Can you work these out from the model? Positions are in its coordinate system, mm. A direction names the side the tool comes from. Coordinates: 2 decimals unless noted, no trailing zeros. Loops run counter-clockwise (first coordinate to the right, second up) from the corner with the lowest first, then second, coordinate; pieces in that order, holes last. Notation, with made-up numbers: (80.25, 69.5) -> (132.25, 69.5) arc R23 ccw to (132.25, 108.5) -> close; hole circle Ø11 at (7.5, -19.75). An arc over 180 degrees is marked (long way). Use one line per item in the form item = value. Start each with the question number.
(1) Imagine slicing it at A-A (x = 0). List the corners of the cut face in (y, z) for me, plus the area to 3 significant figures.
(2) Imagine slicing it at B-B (z = 5). List the corners of the cut face in (x, y) for me.
(3) I need wall thicknesses on line 1 (X direction, y = -6.5, z = 33); line 2 (Z direction, x = 9.25, y = 2); line 3 (Y direction, x = -5, z = 25.5) (3 decimals). Which ranges of each line are inside material? Lowest first, please. Write a range as [from, to].
(4) On a 3-axis mill with a long thin cutter (end or side, diameter ignored), from which of +Z, -Z, +X, -X, +Y, -Y can I reach the whole of each face in a straight line? I mean faces 5 (the flat face through (-2, -9, 38)), 6 (the flat face through (-4, 8, 38)), 7 (the cylindrical face through (5.094, 7.438, 46.381)). Say none if no direction works.
(5) I'm going to push flat-ended pins straight in: pin 1 (2.5 mm diameter, centred on x = 9, y = -2.5, fed in from -Z); pin 2 (4 mm diameter, centred on y = -7.5, z = 5.5, fed in from -X); pin 3 (3 mm diameter, centred on x = 5, z = 23.5, fed in from +Y). Where does each tip first touch, or does it pass through?
(6) Thinking about a two-plate mould opening in X: for faces 1 (the flat face through (4.6, 8.79, 46.38)), 2 (the flat face through (0, 9, 38)), 3 (the cylindrical face through (-6.726, -6.003, 46.381)), 4 (the cylindrical face through (-1.1, -8.9, 46.4)), which applies, released by +X, released by -X, zero draft, split by the parting line, or undercut?
```python
from build123d import *

# Parameters (mm, degrees)
SKETCH1_R           = 8
BOSS_EXTRUDE1_DEPTH = 55
BOSS_EXTRUDE2_START = -17
BOSS_EXTRUDE2_DEPTH = 17
CIRPATTERN1_COUNT   = 13


with BuildPart() as part:
    # Sketch1 → Boss-Extrude1 (new body)
    with BuildSketch(Plane.XY):
        Circle(SKETCH1_R)
    extrude(amount=BOSS_EXTRUDE1_DEPTH)

    # Sketch2 → Boss-Extrude2 (add)
    with BuildSketch(Plane.XY.offset(55).offset(BOSS_EXTRUDE2_START)):
        with BuildLine():
            Line((-0.787121101, 9.92163467), (0.787121101, 9.92163467))
            ThreePointArc((0.787121101, 9.92163467), (1.056170344, 8.938993112), (1.115168142, 7.921893714))
            ThreePointArc((1.115168142, 7.921893714), (0, 8), (-1.115168142, 7.921893714))
            ThreePointArc((-1.115168142, 7.921893714), (-1.056170344, 8.938993112), (-0.787121101, 9.92163467))
        make_face()
    boss_extrude2 = extrude(amount=BOSS_EXTRUDE2_DEPTH)

    # CirPattern1: Boss-Extrude2 ×13 about axis
    cirpattern1_axis = Axis((0, 0, 0), (0, 0, 1))
    for i in range(1, CIRPATTERN1_COUNT):
        add(boss_extrude2.rotate(cirpattern1_axis, i * 360 / CIRPATTERN1_COUNT))


solid = part.part
```
Worked out:
q1.outline = (-8, 0) -> (8, 0) -> (8, 38) -> (9.92, 38) -> (9.92, 55) -> (-8, 55) -> close
q1.area = 913 mm2
q2.outline = circle Ø16 at (0, 0)
q3.line_1 = [-4.66, 4.66]
q3.line_2 = [38, 55]
q3.line_3 = [-6.245, 6.245]
q4.face_5 = -Z, -X, -Y
q4.face_6 = -Z, -X, +Y
q4.face_7 = +Z, -Z, +X
q5.pin_1 = 38
q5.pin_2 = -5.81
q5.pin_3 = 7.19
q6.face_1 = released by +X
q6.face_2 = zero draft
q6.face_3 = released by -X
q6.face_4 = undercut
